Model file for the job. Use its own axes, mm. Face numbers are marked on the shaded views. A direction names the side the tool comes from. Coordinates: 2 decimals unless noted, no trailing zeros. Order: outer loops, then holes, each group sorted by start corner. A loop starts at its lowest first (then second) coordinate and runs counter-clockwise, first axis right, second up. Notation, with made-up numbers: (86.5, 39.25) -> (136.5, 39.25) arc R25 cw to (136.5, 62.25) -> close; hole circle Ø3 at (0.5, -27.75). An arc over 180 degrees is marked (long way). Return JSON: item names as keys, results as strings. Group by question number.
1) Which spindle directions (+Z, -Z, +X, -X, +Y, -Y) get a long thin tool onto all of the face, cutting with end or side? Do the marked faces 1, 2 and 3. Say none if no direction does.
2) Flat gauge pins, fed straight in: pin 1 (7.5 mm diameter, centred on y = -4, z = -7, fed in from +X); pin 2 (7.5 mm diameter, centred on y = 8, z = -4.5, fed in from -X); pin 3 (11.5 mm diameter, centred on x = 186, y = 5.5, fed in from -Z). Where does each tip first touch, or does it go through?
3) Probe line 1 (Z direction, x = 176, y = -3) (3 decimals); line 2 (X direction, y = 18.5, z = -4.5). List the from-to ranges inside material, lowest first.
4) Cut at B-B (z = -4). Write the cut outline in (x, y), and give its area (3 significant figures).
5) Cut at A-A (y = -5). Write the cut outline in (x, z) (3 decimals), and give its area (3 significant figures).
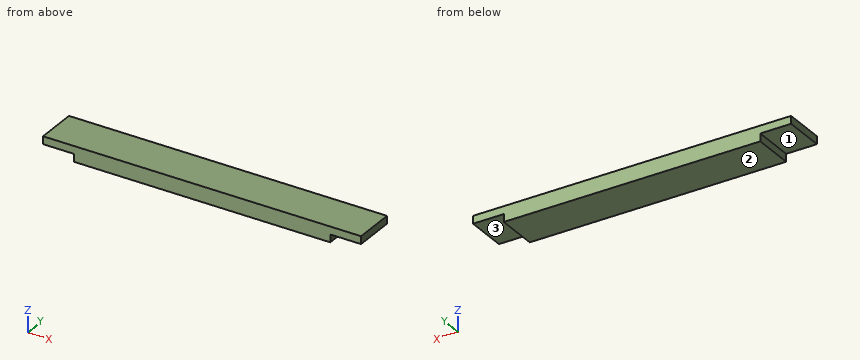
from build123d import *

# Parameters (mm, degrees)
F0_W     = 393.7
F0_H     = 50.8
F1_DEPTH = 9.525
F2_W     = 38.1
F2_H     = 50.8
F3_DEPTH = 9.526


with BuildPart() as f1:
    # F0 (on Top) → F1 (new body, symmetric)
    with BuildSketch(Plane.XY):
        Rectangle(F0_W, F0_H)
    extrude(amount=F1_DEPTH, both=True)

    # F2 (on Top) → F3 (cut, through all)
    with BuildSketch(Plane.XY):
        with Locations((-177.8, 0)):
            Rectangle(F2_W, F2_H)
        with Locations((177.8, 0)):
            Rectangle(F2_W, F2_H)
    extrude(amount=-F3_DEPTH, mode=Mode.SUBTRACT)


solid = f1.part
Answers below:
{
 "1": {"face 1": "-Z, -X, +Y, -Y", "face 2": "-Z, +X, -X, +Y, -Y", "face 3": "-Z, +X, +Y, -Y"},
 "2": {"pin 1": "stops at x = 158.75", "pin 2": "stops at x = -158.75", "pin 3": "stops at z = 0"},
 "3": {"line 1": "z = 0 to 9.525", "line 2": "x = -158.75 to 158.75"},
 "4": {"outline": "(-158.75, -25.4) -> (158.75, -25.4) -> (158.75, 25.4) -> (-158.75, 25.4) -> close", "area": "16,100 mm^2"},
 "5": {"outline": "(-196.85, 0) -> (-158.75, 0) -> (-158.75, -9.525) -> (158.75, -9.525) -> (158.75, 0) -> (196.85, 0) -> (196.85, 9.525) -> (-196.85, 9.525) -> close", "area": "6,770 mm^2"}
}
